Autodesk Inventor part; units mm, degrees
ref_plane "Plano de trabajo1" through (0, 0, 0) normal (0, 0, 1) x (1, 0, 0)
ref_plane "YZ Plane" through (0, 0, 0) normal (1, 0, 0) x (0, 1, 0)
ref_plane "XZ Plane" through (0, 0, 0) normal (0, 1, 0) x (-1, 0, 0)
ref_plane "Plano de trabajo1" through (0, 0, 0) normal (0, 0, 1) x (1, 0, 0)
sketch "Boceto1" plane through (0, 0, 0) normal (0, 0, 1) x (1, 0, 0)
  line L0 (50.85, -50.85) -> (50.85, 50.85)
  line L1 (50.85, 50.85) -> (-50.85, 50.85)
  line L2 (-50.85, 50.85) -> (-50.85, -50.85)
  line L3 (-50.85, -50.85) -> (50.85, -50.85)
  circle A0 centre (-40.8484, 40.8516) radius 2.8882
  circle A1 centre (40.8516, 40.8516) radius 2.5
  circle A2 centre (-40.8484, -40.8484) radius 2.8882
  circle A3 centre (40.8516, -40.8484) radius 2.5
  point P0 (0, 0)
extrude "Extrusión1" add sketch "Boceto1" along normal blind 1.65
sketch "Boceto2" plane through (0, 0, 1.65) normal (0, 0, 1) x (1, 0, 0)
  line L0 (14.2817, 24.0293) -> (-14.2817, 24.0293)
  line L1 (-14.2817, 24.0293) -> (-14.2817, -24.0293)
  line L2 (-14.2817, -24.0293) -> (14.2817, -24.0293)
  line L3 (14.2817, -24.0293) -> (14.2817, 24.0293)
  line L4 (14.2817, 24.0293) -> (-14.2817, -24.0293) construction
  line L5 (-14.2817, 24.0293) -> (14.2817, -24.0293) construction
  point P0 (0, 0)
extrude "Extrusión2" add sketch "Boceto2" along normal blind 18.5
sketch "Boceto3" plane through (0, 0, 20.15) normal (0, 0, 1) x (1, 0, 0)
  circle A0 centre (0, 0) radius 4.3846
extrude "Extrusión3" add sketch "Boceto3" along normal blind 5
sketch "Boceto4" plane through (0, 0, 25.15) normal (0, 0, 1) x (1, 0, 0)
  circle A0 centre (0, 0) radius 26.7
  dimension "d6" = 53.4
extrude "Extrusión4" add sketch "Boceto4" along normal blind 27
sketch "Boceto5" plane through (0, 0, 52.15) normal (0, 0, 1) x (1, 0, 0)
  circle A0 centre (0, 0) radius 4.3846
extrude "Extrusión5" add sketch "Boceto5" along normal blind 5
properties part number "PCB_RW"
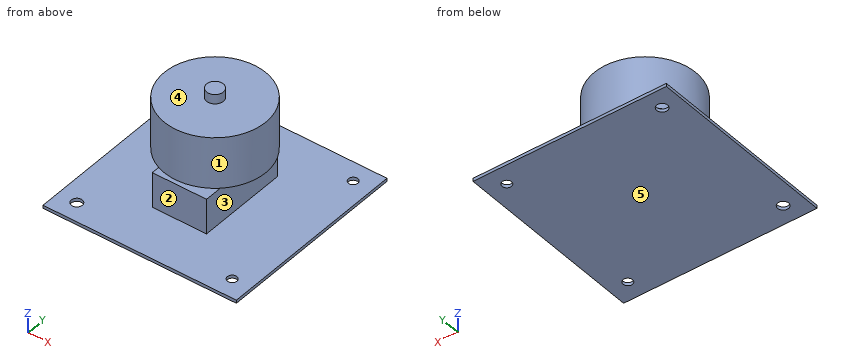
Build history of the part. All positions in model axes, mm. Face numbers are marked on the shaded views. A direction names the side the tool comes from. Round coordinates to 2 decimals unless told otherwise and drop trailing zeros. Write each loop counter-clockwise with the first axis right and the second up, starting at its lowest first coordinate (ties: lowest second). Pieces come first, ordered by that corner, then holes. Notation, with made-up numbers: M 68,56 L 111,56 A29 ccw 111,86 Z; hole C 65,8 d3. An arc over 180 degrees is marked long. Answer in a Markdown table with one row per item.
1. Mould opens along Z. For the marked faces 3, 4 and 5 say: +Z half, -Z half, draft (parallel to the pull), parting line (faces both ways), or undercut.
Geometry check:
| item | result |
|---|---|
| face 3 | undercut |
| face 4 | +Z half |
| face 5 | -Z half |
2. Saw through at A-A (y = 0). List the corners of the cut face in (x, z), and give its area (3 significant figures).
Geometry check:
| item | result |
|---|---|
| outline | M -50.85,0 L 50.85,0 L 50.85,1.65 L 14.28,1.65 L 14.28,20.15 L 4.38,20.15 L 4.38,25.15 L 26.7,25.15 L 26.7,52.15 L 4.38,52.15 L 4.38,57.15 L -4.38,57.15 L -4.38,52.15 L -26.7,52.15 L -26.7,25.15 L -4.38,25.15 L -4.38,20.15 L -14.28,20.15 L -14.28,1.65 L -50.85,1.65 Z |
| area | 2,230 mm2 |
3. Flat gauge pins, fed straight in: P1, Ø15, axis at y = -10.5, z = 10, coming from the +X side; P2, Ø6.5, axis at x = 40.85, y = 40.85, coming from the +Z side; P3, Ø20.5, axis at x = 3.5, z = 13.5, coming from the -Y side; P4, Ø4.5, axis at x = 40.85, y = -40.85, coming from the -Z side. Where does each tip first touch, or does it go through?
Geometry check:
| item | result |
|---|---|
| P1 | x = 14.28 |
| P2 | z = 1.65 |
| P3 | y = -24.03 |
| P4 | through |
4. Saw through at B-B (x = -17). List the corners of the cut face in (y, z), and give its area (3 significant figures).
Geometry check:
| item | result |
|---|---|
| outline | M -50.85,0 L 50.85,0 L 50.85,1.65 L -50.85,1.65 Z; M -20.59,25.15 L 20.59,25.15 L 20.59,52.15 L -20.59,52.15 Z |
| area | 1,280 mm2 |
5. Which spindle directions (+Z, -Z, +X, -X, +Y, -Y) get a long thin tool onto all of the face, cutting with end or side? Do the marked faces 1 and 2. Say none if no direction does.
Geometry check:
| item | result |
|---|---|
| face 1 | +Z |
| face 2 | +X, -X, -Y |
6. Saw through at D-D (x = 0). List the corners of the cut face in (y, z).
Geometry check:
| item | result |
|---|---|
| outline | M -50.85,0 L 50.85,0 L 50.85,1.65 L 24.03,1.65 L 24.03,20.15 L 4.38,20.15 L 4.38,25.15 L 26.7,25.15 L 26.7,52.15 L 4.38,52.15 L 4.38,57.15 L -4.38,57.15 L -4.38,52.15 L -26.7,52.15 L -26.7,25.15 L -4.38,25.15 L -4.38,20.15 L -24.03,20.15 L -24.03,1.65 L -50.85,1.65 Z |
7. Probe L1, parallel to Z at x = 18, y = 0.5; L2, parallel to Z at x = 6, y = -19; L3, parallel to Y at x = 13.5, z = 15.5. List the from-to ranges inside material, lowest first. Write a range as [from, to].
Geometry check:
| item | result |
|---|---|
| L1 | [0, 1.65], [25.15, 52.15] |
| L2 | [0, 20.15], [25.15, 52.15] |
| L3 | [-24.03, 24.03] |
8. Saw through at C-C (y = -14). List the corners of the cut face in (x, z), and give its area (3 significant figures).
Geometry check:
| item | result |
|---|---|
| outline | M -50.85,0 L 50.85,0 L 50.85,1.65 L 14.28,1.65 L 14.28,20.15 L -14.28,20.15 L -14.28,1.65 L -50.85,1.65 Z; M -22.74,25.15 L 22.74,25.15 L 22.74,52.15 L -22.74,52.15 Z |
| area | 1,920 mm2 |
